The listing builds one solid part. Answer for the finished solid, in the listing's coordinates (mm). A direction names the side the tool comes from. Round coordinates to 2 decimals unless told otherwise and drop trailing zeros. Write each loop counter-clockwise with the first axis right and the second up, starting at its lowest first coordinate (ties: lowest second). Pieces come first, ordered by that corner, then holes. Notation, with made-up numbers: M 4,44 L 60,44 A25 ccw 60,73 Z; hole C 78.25,56 d2. An arc over 180 degrees is marked long. Write each question's results on one line, items separated by ' | '.
from build123d import *

# Parameters (mm, degrees)
SKETCH1_W           = 56.4
SKETCH1_H           = 56.4
BOSS_EXTRUDE1_DEPTH = 56
SKETCH2_R           = 2.5
CUT_EXTRUDE1_DEPTH  = 56
CUT_EXTRUDE2_DEPTH  = 51
FILLET1_R           = 5
SKETCH5_R           = 19.05
BOSS_EXTRUDE2_DEPTH = 1.6
SKETCH6_R           = 3.175
BOSS_EXTRUDE3_DEPTH = 19.6
CUT_EXTRUDE3_START  = -17
CUT_EXTRUDE3_DEPTH  = 17


with BuildPart() as part:
    # Sketch1 → Boss-Extrude1 (new body)
    with BuildSketch(Plane(origin=(0, 0, 0), x_dir=(1, 0, 0), z_dir=(0, 1, 0))):
        Rectangle(SKETCH1_W, SKETCH1_H)
    extrude(amount=BOSS_EXTRUDE1_DEPTH)

    # Sketch2 → Cut-Extrude1 (cut)
    with BuildSketch(Plane(origin=(0, 56, 0), x_dir=(1, 0, 0), z_dir=(0, 1, 0))):
        with Locations(Location((-23.57, 23.57, 0), (0, 0, 270))):
            Circle(SKETCH2_R)
        with Locations(Location((23.57, 23.57, 0), (0, 0, 270))):
            Circle(SKETCH2_R)
        with Locations(Location((23.57, -23.57, 0), (0, 0, 270))):
            Circle(SKETCH2_R)
        with Locations(Location((-23.57, -23.57, 0), (0, 0, 270))):
            Circle(SKETCH2_R)
    extrude(amount=-CUT_EXTRUDE1_DEPTH, mode=Mode.SUBTRACT)

    # Sketch4 → Cut-Extrude2 (cut)
    with BuildSketch(Plane.XZ):
        with BuildLine():
            Line((-18.57, 23.57), (-18.57, 28.2))
            Line((-18.57, 28.2), (-28.2, 28.2))
            Line((-28.2, 28.2), (-28.2, 18.57))
            Line((-28.2, 18.57), (-23.57, 18.57))
            ThreePointArc((-23.57, 18.57), (-20.034466094, 20.034466094), (-18.57, 23.57))
        make_face()
        with BuildLine():
            Line((23.57, 18.57), (28.2, 18.57))
            Line((28.2, 18.57), (28.2, 28.2))
            Line((28.2, 28.2), (18.57, 28.2))
            Line((18.57, 28.2), (18.57, 23.57))
            ThreePointArc((18.57, 23.57), (20.034466094, 20.034466094), (23.57, 18.57))
        make_face()
        with BuildLine():
            Line((18.57, -23.57), (18.57, -28.2))
            Line((18.57, -28.2), (28.2, -28.2))
            Line((28.2, -28.2), (28.2, -18.57))
            Line((28.2, -18.57), (23.57, -18.57))
            ThreePointArc((23.57, -18.57), (20.034466094, -20.034466094), (18.57, -23.57))
        make_face()
        with BuildLine():
            Line((-23.57, -18.57), (-28.2, -18.57))
            Line((-28.2, -18.57), (-28.2, -28.2))
            Line((-28.2, -28.2), (-18.57, -28.2))
            Line((-18.57, -28.2), (-18.57, -23.57))
            ThreePointArc((-18.57, -23.57), (-20.034466094, -20.034466094), (-23.57, -18.57))
        make_face()
    extrude(amount=-CUT_EXTRUDE2_DEPTH, mode=Mode.SUBTRACT)

    # Fillet1
    fillet1_edges = [part.edges().sort_by_distance(p)[0] for p in [
        (28.2, 53.5, 28.2),
        (-28.2, 53.5, 28.2),
        (-28.2, 53.5, -28.2),
        (28.2, 53.5, -28.2),
    ]]
    fillet(fillet1_edges, radius=FILLET1_R)

    # Sketch5 → Boss-Extrude2 (add)
    with BuildSketch(Plane(origin=(0, 56, 0), x_dir=(1, 0, 0), z_dir=(0, 1, 0))):
        with Locations(Location((0, 0, 0), (0, 0, 90))):
            Circle(SKETCH5_R)
    extrude(amount=BOSS_EXTRUDE2_DEPTH)

    # Sketch6 → Boss-Extrude3 (add)
    with BuildSketch(Plane(origin=(0, 57.6, 0), x_dir=(1, 0, 0), z_dir=(0, 1, 0))):
        with Locations(Location((0, 0, 0), (0, 0, 270))):
            Circle(SKETCH6_R)
    extrude(amount=BOSS_EXTRUDE3_DEPTH)

    # Sketch7 → Cut-Extrude3 (cut)
    with BuildSketch(Plane(origin=(0, 77.2, 0), x_dir=(1, 0, 0), z_dir=(0, 1, 0)).offset(CUT_EXTRUDE3_START)):
        with BuildLine():
            Line((-1.963568181, 2.495), (1.963568181, 2.495))
            ThreePointArc((1.963568181, 2.495), (0, 3.175), (-1.963568181, 2.495))
        make_face()
    extrude(amount=CUT_EXTRUDE3_DEPTH, mode=Mode.SUBTRACT)


solid = part.part
1) The mould has two halves that part along Z. Classify faces 1 (the face through (-28.2, 28, 0)), 2 (the face through (0, 28, 28.2)), 3 (the face through (0.95, 67.26, 3.03)), 4 (the face through (25.26, 53.54, 21.73)): +Z half, -Z half, draft (parallel to the pull), parting line (faces both ways), or undercut.
Return value:
face 1: draft | face 2: +Z half | face 3: parting line | face 4: undercut
2) Section C-C (z = -1) is taken. Determine the outline of the cut face in (x, y), then the cut area to 3 significant figures.
Return value:
outline: M -28.2,0 L 28.2,0 L 28.2,56 L 19.02,56 L 19.02,57.6 L 3.01,57.6 L 3.01,77.2 L -3.01,77.2 L -3.01,57.6 L -19.02,57.6 L -19.02,56 L -28.2,56 Z | area: 3,340 mm²
3) Find the intervals of material crossed by line 1 (X direction, y = 54.65, z = 23.57); line 2 (X direction, y = 53, z = 23); line 3 (Y direction, x = -16.5, z = 1), in increasing order.
Return value:
line 1: -28.19 to -26.07, -21.07 to 21.07, 26.07 to 28.19 | line 2: -28.2 to -26, -21.14 to 21.14, 26 to 28.2 | line 3: 0 to 57.6
4) A tool of negligible diameter and unlimited length cuts with its end or side. For faces 5 (the face through (-18.57, 25, 26)), 6 (the face through (26, 25, -18.57)), 7 (the face through (0, 69, -2.495)), 8 (the face through (21, 51, 22)), 9 (the face through (-26, 25, -18.57)), from which of +Z, -Z, +X, -X, +Y, -Y can it reach the whole face along a straight path? Write none if from no direction.
Return value:
face 5: +Z, -X, -Y | face 6: -Z, +X, -Y | face 7: -Z, +X, -X, +Y | face 8: +Z, +X, -Y | face 9: -Z, -X, -Y
5) Section D-D (z = 15.5) is taken. Determine the outline of the cut face in (x, y), then the cut area to 3 significant figures.
Return value:
outline: M -28.2,0 L 28.2,0 L 28.2,56 L 11.07,56 L 11.07,57.6 L -11.07,57.6 L -11.07,56 L -28.2,56 Z | area: 3,190 mm²
6) Each of these flat-tipped pins is pushed along its axis until it touches: pin 1 (1.5 mm diameter, centred on x = -22.5, z = -15.5, fed in from +Y); pin 2 (5 mm diameter, centred on x = -2, z = -20.5, fed in from -Y); pin 3 (3 mm diameter, centred on x = 23.57, z = -23.57, fed in from -Y); pin 4 (5 mm diameter, centred on x = 23, z = 22, fed in from -Y). Where does it stop, or does it pass through?
Return value:
pin 1: y = 56 | pin 2: y = 0 | pin 3: through | pin 4: y = 51
7) Section A-A (y = 10) is taken. Determine the outline of the cut face in (x, z).
Return value:
outline: M -28.2,-18.57 L -23.57,-18.57 A5 cw -18.57,-23.57 L -18.57,-28.2 L 18.57,-28.2 L 18.57,-23.57 A5 cw 23.57,-18.57 L 28.2,-18.57 L 28.2,18.57 L 23.57,18.57 A5 cw 18.57,23.57 L 18.57,28.2 L -18.57,28.2 L -18.57,23.57 A5 cw -23.57,18.57 L -28.2,18.57 Z
8) Section B-B (x = 11.5) is taken. Determine the outline of the cut face in (y, z), then the cut area to 3 significant figures.
Return value:
outline: M 0,-28.2 L 56,-28.2 L 56,-15.19 L 57.6,-15.19 L 57.6,15.19 L 56,15.19 L 56,28.2 L 0,28.2 Z | area: 3,210 mm²
